Part print with two shaded views. Sizes in mm from the minimum x, y, z corner. A direction names the side the tool comes from. Give positions to 0.01 mm unless a question says otherwise; leave off trailing zeros. Order: outer loops, then holes, each group sorted by start corner. A loop starts at its lowest first (then second) coordinate and runs counter-clockwise, first axis right, second up.
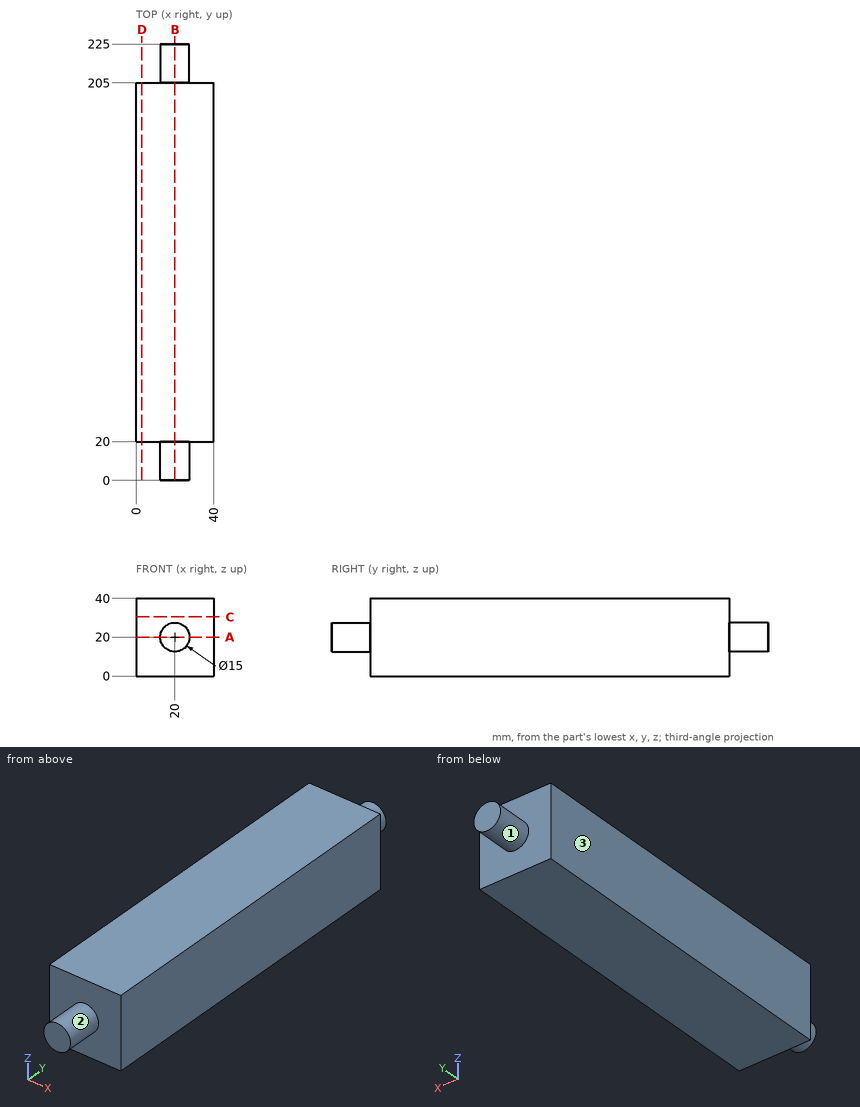
1. Saw through at B-B on x = 20. Give the cut face in (y, z), plus the area to 3 significant figures.
2. Wall check: line 1 (Y direction, x = 7, z = 16). Give the ranges that are in metal, low to high.
3. Saw through at C-C on z = 30.5. Give the cut face in (x, y), plus the area to 3 significant figures.
4. Saw through at D-D on x = 3. Give the cut face in (y, z), plus the area to 3 significant figures.
5. Pin check, flat tips, straight feed: P1, Ø5, axis at x = 11.5, z = 8, coming from the -Y side; P2, Ø10, axis at x = 18.5, z = 36, coming from the +Y side. Stop position of each tip, or through.
6. 3-axis set-ups, long thin cutter, end or side, ignore diameter. For the marked faces 1, 2 and 3: which of +Z, -Z, +X, -X, +Y, -Y reach the whole face in a straight line?
7. Saw through at A-A on z = 20. Give the cut face in (x, y), plus the area to 3 significant figures.
Reported:
1. outline: (0, 12.5) - (20, 12.5) - (20, 0) - (205, 0) - (205, 12.5) - (225, 12.5) - (225, 27.5) - (205, 27.5) - (205, 40) - (20, 40) - (20, 27.5) - (0, 27.5) - close
1. area: 8,000 mm2
2. line 1: y = 20 to 205
3. outline: (0, 20) - (40, 20) - (40, 205) - (0, 205) - close
3. area: 7,400 mm2
4. outline: (20, 0) - (205, 0) - (205, 40) - (20, 40) - close
4. area: 7,400 mm2
5. P1: stops at y = 20
5. P2: stops at y = 205
6. face 1: +Y
6. face 2: -Y
6. face 3: +Z, -Z, -X, +Y, -Y
7. outline: (0, 20) - (12.5, 20) - (12.5, 0) - (27.5, 0) - (27.5, 20) - (40, 20) - (40, 205) - (27.5, 205) - (27.5, 225) - (12.5, 225) - (12.5, 205) - (0, 205) - close
7. area: 8,000 mm2
